Autodesk Inventor part; units mm, degrees
ref_plane "YZ Plane" through (0, 0, 0) normal (1, 0, 0) x (0, 1, 0)
ref_plane "XZ Plane" through (0, 0, 0) normal (0, 1, 0) x (-1, 0, 0)
ref_plane "XY Plane" through (0, 0, 0) normal (0, 0, 1) x (1, 0, 0)
sketch "Sketch1" plane through (0, 0, 0) normal (0, 1, 0) x (-1, 0, 0)
  line L0 (0, 0) -> (22.5, 0)
  line L1 (22.5, 0) -> (22.5, -62)
  line L2 (22.5, -62) -> (0, -62)
  line L3 (0, -62) -> (0, 0)
  dimension "d0" = 22.5
  dimension "d1" = 62
extrude "Extrusion1" add sketch "Sketch1" along normal blind 6.5
sketch "Sketch2" plane through (0, 6.5, 0) normal (0, 1, 0) x (1, 0, 0)
  line L0 (0, 62) -> (-22.5, 62)
  line L1 (-22.5, 62) -> (-22.5, 0)
  circle A0 centre (-16.25, 56.5) radius 1.5
  circle A1 centre (-16.25, 47.5) radius 1.5
  circle A2 centre (-6.25, 56.5) radius 1.5
  circle A3 centre (-6.25, 47.5) radius 1.5
  circle A4 centre (-16.25, 14.5) radius 1.5
  circle A5 centre (-16.25, 5.5) radius 1.5
  circle A6 centre (-6.25, 14.5) radius 1.5
  circle A7 centre (-6.25, 5.5) radius 1.5
  line L2 (-16.25, 56.5) -> (-6.25, 56.5) construction
  line L3 (-16.25, 56.5) -> (-6.25, 47.5) construction
  line L4 (-16.25, 47.5) -> (-6.25, 56.5) construction
  line L5 (-16.25, 14.5) -> (-6.25, 5.5) construction
  line L6 (-6.25, 14.5) -> (-16.25, 5.5) construction
  line L7 (-11.25, 52) -> (-11.25, 10) construction
  point P0 (-11.25, 56.5)
  point P1 (-11.25, 62)
  point P2 (-11.25, 31)
  point P3 (-22.5, 31)
  dimension "d5" = 3
  dimension "d6" = 9
  dimension "d7" = 10
  dimension "d8" = 9
  dimension "d9" = 42
extrude "Extrusion2" cut sketch "Sketch2" against normal through all
equation "\"d8\" = d6"
properties part number "x_iddler_right_cap"
Check sheet for the modelled part. Datum: model origin and axes. Units: mm. Give positions to 0.01 mm unless a question says otherwise; leave off trailing zeros. Write each loop counter-clockwise with the first axis right and the second up, starting at its lowest first coordinate (ties: lowest second). Pieces come first, ordered by that corner, then holes. Notation, with made-up numbers: (54, 79) -> (74, 79) arc R21 cw to (74, 118) -> close; hole circle Ø1 at (75, 27). An arc over 180 degrees is marked (long way). Use one line per item in the form item = value. Start each with the question number.
1. Section check D-D (x = -5.5). Record the cut outline in (y, z).
2. Section check A-A (x = -16.25). Record the cut outline in (y, z).
3. Section check C-C (z = -14.5). Record the cut outline in (x, y).
4. Section check B-B (y = 2.5). Count the separate pieces of the cut face and the enclosed holes in it, and give its area (3 significant figures).
5. Go/stop test with a flat-tipped pin: P1, Ø2.5, axis at x = -6.25, z = -14.5, coming from the +Y side. Record where the tip stops, or that it passes through.
6. Mould release check, pull along Z, two halves, no side actions. Record for faces 1 (the flat face through (-11, 3, 0)), 2 (the flat face through (-11, 6.5, -31)), 3 (the flat face through (-11, 3, -62)), 4 (the cylindrical face through (-6.575, 3.296, -46.036)): pulls with the +Z half, pulls with the -Z half, needs draft (parallel to the pull), parting line crosses it, or undercut.
7. Thickness scan on line 1 along X through (y, z) = (3.75, -5.5); line 2 along Z through (x, y) = (-16.25, 3); line 3 along Z through (x, y) = (-15.75, 4.5). Record the ranges inside material, lowest first. Write a range as from..to.
Conclusion:
q1.outline = (0, -62) -> (6.5, -62) -> (6.5, -57.8) -> (0, -57.8) -> close; (0, -55.2) -> (6.5, -55.2) -> (6.5, -48.8) -> (0, -48.8) -> close; (0, -46.2) -> (6.5, -46.2) -> (6.5, -15.8) -> (0, -15.8) -> close; (0, -13.2) -> (6.5, -13.2) -> (6.5, -6.8) -> (0, -6.8) -> close; (0, -4.2) -> (6.5, -4.2) -> (6.5, 0) -> (0, 0) -> close
q2.outline = (0, -62) -> (6.5, -62) -> (6.5, -58) -> (0, -58) -> close; (0, -55) -> (6.5, -55) -> (6.5, -49) -> (0, -49) -> close; (0, -46) -> (6.5, -46) -> (6.5, -16) -> (0, -16) -> close; (0, -13) -> (6.5, -13) -> (6.5, -7) -> (0, -7) -> close; (0, -4) -> (6.5, -4) -> (6.5, 0) -> (0, 0) -> close
q3.outline = (-22.5, 0) -> (-17.75, 0) -> (-17.75, 6.5) -> (-22.5, 6.5) -> close; (-14.75, 0) -> (-7.75, 0) -> (-7.75, 6.5) -> (-14.75, 6.5) -> close; (-4.75, 0) -> (0, 0) -> (0, 6.5) -> (-4.75, 6.5) -> close
q4.separate_pieces = 1
q4.enclosed_holes = 8
q4.area = 1,340 mm²
q5.P1 = through
q6.face_1 = pulls with the +Z half
q6.face_2 = needs draft
q6.face_3 = pulls with the -Z half
q6.face_4 = undercut
q7.line_1 = -22.5..-17.75, -14.75..-7.75, -4.75..0
q7.line_2 = -62..-58, -55..-49, -46..-16, -13..-7, -4..0
q7.line_3 = -62..-57.91, -55.09..-48.91, -46.09..-15.91, -13.09..-6.91, -4.09..0
